from build123d import *

# Parameters (mm, degrees)
SKETCH_1_R      = 12
SKETCH_1_R_2    = 9
EXTRUDE_1_DEPTH = 3
SKETCH_2_R      = 9
SKETCH_2_R_2    = 1.5
EXTRUDE_2_DEPTH = 3


with BuildPart() as part:
    # 草图1 → 凸台-拉伸1 (new body)
    with BuildSketch(Plane(origin=(0, 0, 0), x_dir=(1, 0, 0), z_dir=(0, 1, 0))):
        with Locations(Location((0, 0, 0), (0, 0, 270))):
            Circle(SKETCH_1_R)
        with Locations(Location((0, 0, 0), (0, 0, 270))):
            Circle(SKETCH_1_R_2, mode=Mode.SUBTRACT)
    extrude(amount=EXTRUDE_1_DEPTH)

    # 草图2 → 凸台-拉伸2 (add)
    with BuildSketch(Plane(origin=(0, 3, 0), x_dir=(1, 0, 0), z_dir=(0, 1, 0))):
        with BuildLine():
            Line((-10, -11.180339887), (-10, -20))
            Line((-10, -20), (10, -20))
            Line((10, -20), (10, -11.180339887))
            ThreePointArc((10, -11.180339887), (15, 0), (10, 11.180339887))
            Line((10, 11.180339887), (10, 20))
            Line((10, 20), (-10, 20))
            Line((-10, 20), (-10, 11.180339887))
            ThreePointArc((-10, 11.180339887), (-15, 0), (-10, -11.180339887))
        make_face()
        with Locations(Location((0, 0, 0), (0, 0, 270))):
            Circle(SKETCH_2_R, mode=Mode.SUBTRACT)
        with Locations(Location((-5, 16, 0), (0, 0, 270))):
            Circle(SKETCH_2_R_2, mode=Mode.SUBTRACT)
        with Locations(Location((5, 16, 0), (0, 0, 270))):
            Circle(SKETCH_2_R_2, mode=Mode.SUBTRACT)
        with Locations(Location((-5, -16, 0), (0, 0, 270))):
            Circle(SKETCH_2_R_2, mode=Mode.SUBTRACT)
        with Locations(Location((5, -16, 0), (0, 0, 270))):
            Circle(SKETCH_2_R_2, mode=Mode.SUBTRACT)
    extrude(amount=EXTRUDE_2_DEPTH)


solid = part.part
The model under review builds one solid part; all positions refer to its coordinate system, in mm. A direction names the side the tool comes from. Coordinates: 2 decimals unless noted, no trailing zeros. Write each loop counter-clockwise with the first axis right and the second up, starting at its lowest first coordinate (ties: lowest second). Pieces come first, ordered by that corner, then holes. Notation, with made-up numbers: (41, -29.5) - (59, -29.5) arc R26 ccw to (59, -1.5) - close; hole circle Ø5 at (19.5, 77). An arc over 180 degrees is marked (long way). Answer as a JSON object with one key per item and string values. Group by question number.
1. Add section A-A (z = 0). Give the boundary of the cut face in (x, y), plus the area to 3 significant figures.
2. Machinability: for faces 4 (the face through (-10, 4, 16)), 5 (the face through (5.07, 4.48, -17.5)), 6 (the face through (-10, 4, -16)), 7 (the face through (10, 4, -16)), 8 (the face through (13, 3, 0)), which of the approach directions +Z, -Z, +X, -X, +Y, -Y give a long, thin tool a straight path to every point of the face, cutting with its end or side? Answer none if there is none.
3. Add section D-D (z = -16). Give the boundary of the cut face in (x, y).
4. Mouldability with a two-part tool opening along Z and no side actions: class faces 1 (the face through (-4.93, 4.48, -17.5)), 2 (the face through (10, 4, 16)), 3 (the face through (0, 4, -20)) as pulls with the +Z half, pulls with the -Z half, needs draft (parallel to the pull), parting line crosses it, or undercut.
5. Add section B-B (x = 0). Give the boundary of the cut face in (y, z), plus the area to 3 significant figures.
6. To check wall thickness, follow probe 1 along X at (y, z) = (5.1, -16); probe 2 along X at (y, z) = (3.2, 15); probe 3 along Y at (x, z) = (13.25, 4). State the ranges of each line that lie inside material, in increasing order.
7. Clearance check with flat-ended pins moving along their axes: pin 1 Ø5 at (x, z) = (-5, -16) entering from -Y; pin 2 Ø1 at (x, y) = (1, 1.5) entering from +Z; pin 3 Ø1.5 at (y, z) = (4.5, -15) entering from -X; pin 4 Ø2.5 at (x, z) = (-5, 16) entering from +Y. State where each tip first meets the part, or that it passes through.
8. Add section C-C (y = 5.05). Give the boundary of the cut face in (x, z), plus the area to 3 significant figures.
Findings:
{
 "1": {"outline": "(-15, 3) - (-12, 3) - (-12, 0) - (-9, 0) - (-9, 6) - (-15, 6) - close; (9, 0) - (12, 0) - (12, 3) - (15, 3) - (15, 6) - (9, 6) - close", "area": "54.0 mm²"},
 "2": {"face 4": "+Z, -X, +Y, -Y", "face 5": "+Y, -Y", "face 6": "-Z, -X, +Y, -Y", "face 7": "-Z, +X, +Y, -Y", "face 8": "-Y"},
 "3": {"outline": "(-10, 3) - (-6.5, 3) - (-6.5, 6) - (-10, 6) - close; (-3.5, 3) - (3.5, 3) - (3.5, 6) - (-3.5, 6) - close; (6.5, 3) - (10, 3) - (10, 6) - (6.5, 6) - close"},
 "4": {"face 1": "undercut", "face 2": "needs draft", "face 3": "pulls with the -Z half"},
 "5": {"outline": "(0, -12) - (3, -12) - (3, -20) - (6, -20) - (6, -9) - (0, -9) - close; (0, 9) - (6, 9) - (6, 20) - (3, 20) - (3, 12) - (0, 12) - close", "area": "84.0 mm²"},
 "6": {"probe 1": "-10 to -6.5, -3.5 to 3.5, 6.5 to 10", "probe 2": "-10 to -6.12, -3.88 to 3.88, 6.12 to 10", "probe 3": "3 to 6"},
 "7": {"pin 1": "y = 3", "pin 2": "z = 11.99", "pin 3": "x = -10", "pin 4": "through"},
 "8": {"outline": "(-10, -20) - (10, -20) - (10, -11.18) arc R15 ccw to (10, 11.18) - (10, 20) - (-10, 20) - (-10, 11.18) arc R15 ccw to (-10, -11.18) - close; hole circle Ø18 at (0, 0); hole circle Ø3 at (-5, -16); hole circle Ø3 at (-5, 16); hole circle Ø3 at (5, -16); hole circle Ø3 at (5, 16)", "area": "672 mm²"}
}
